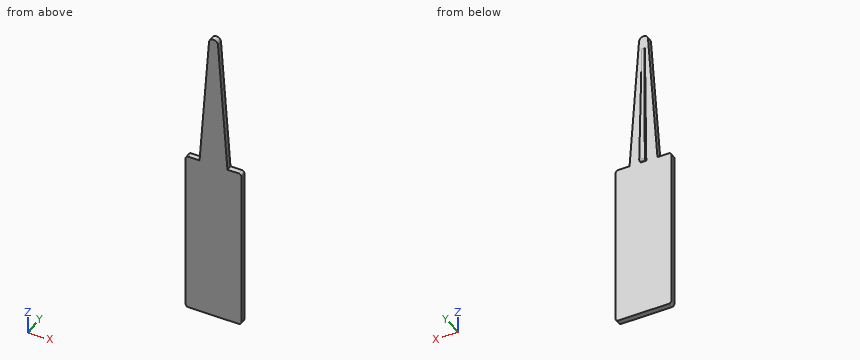
from build123d import *

# Parameters (mm, degrees)
BOSS_EXTRUDE1_DEPTH = 2
FILLET2_R           = 1
FILLET3_R           = 1
FILLET4_R           = 1
FILLET5_R           = 1
BOSS_EXTRUDE2_DEPTH = 1
DRAFT1_ANGLE        = -1
FILLET7_R           = 0.5


with BuildPart() as part:
    # Sketch1 → Boss-Extrude1 (new body)
    with BuildSketch(Plane(origin=(0, 0, 0), x_dir=(1, 0, 0), z_dir=(0, 1, 0))):
        with BuildLine():
            Line((0, 0), (20, 0))
            Line((20, 0), (20, -60))
            Line((20, -60), (15, -60))
            Line((15, -60), (11.6, -108.508220533))
            ThreePointArc((11.6, -108.508220533), (10, -110), (8.4, -108.508220533))
            Line((8.4, -108.508220533), (5, -60))
            Line((5, -60), (0, -60))
            Line((0, -60), (0, 0))
        make_face()
    extrude(amount=BOSS_EXTRUDE1_DEPTH)

    # Fillet2
    fillet2_edges = [part.edges().sort_by_distance(p)[0] for p in [
        (0, 1, 0),
    ]]
    fillet(fillet2_edges, radius=FILLET2_R)

    # Fillet3
    fillet3_edges = [part.edges().sort_by_distance(p)[0] for p in [
        (20, 1, 60),
    ]]
    fillet(fillet3_edges, radius=FILLET3_R)

    # Fillet4
    fillet4_edges = [part.edges().sort_by_distance(p)[0] for p in [
        (20, 1, 0),
    ]]
    fillet(fillet4_edges, radius=FILLET4_R)

    # Fillet5
    fillet5_edges = [part.edges().sort_by_distance(p)[0] for p in [
        (0, 1, 60),
    ]]
    fillet(fillet5_edges, radius=FILLET5_R)

    # Sketch5 → Boss-Extrude2 (add)
    with BuildSketch(Plane(origin=(0, 2, 0), x_dir=(1, 0, 0), z_dir=(0, 1, 0))):
        Polygon((11, -60), (9, -60), (9.5, -105), (10.5, -105), align=None)
    extrude(amount=BOSS_EXTRUDE2_DEPTH)

    # Draft1
    draft1_faces = [part.faces().sort_by_distance(p)[0] for p in [
        (10, 3, 80),
    ]]
    draft(draft1_faces, Plane(origin=(11, 3, 60), x_dir=(-1, 0, 0), z_dir=(0, 0, -1)), DRAFT1_ANGLE)

    # Fillet7
    fillet7_edges = [part.edges().sort_by_distance(p)[0] for p in [
        (10, 3, 60),
    ]]
    fillet(fillet7_edges, radius=FILLET7_R)


solid = part.part
Read the model definition and answer for the solid it produces. Units are mm, in the model's axes. Give positions to 0.01 mm unless a question says otherwise; leave off trailing zeros. Write each loop counter-clockwise with the first axis right and the second up, starting at its lowest first coordinate (ties: lowest second). Pieces come first, ordered by that corner, then holes. Notation, with made-up numbers: (88.5, 9.5) - (108.5, 9.5) arc R23 cw to (108.5, 48.5) - close; hole circle Ø10 at (-10.5, -17.75). An arc over 180 degrees is marked (long way). Return JSON: item names as keys, results as strings.
Q1. A cutting plane is placed at B-B, the plane z = 55. Determine the outline of the cut face in (x, y), and give its area (3 significant figures).
Reply:
{"outline": "(0, 0) - (20, 0) - (20, 2) - (0, 2) - close", "area": "40.0 mm²"}
Q2. A cutting plane is placed at A-A, the plane y = 0.9. Determine the outline of the cut face in (x, z).
Reply:
{"outline": "(0, 1) arc R1 ccw to (1, 0) - (19, 0) arc R1 ccw to (20, 1) - (20, 59) arc R1 ccw to (19, 60) - (15, 60) - (11.6, 108.51) arc R1.6 ccw to (8.4, 108.51) - (5, 60) - (1, 60) arc R1 ccw to (0, 59) - close"}
Q3. Consider line 1 along Y through (x, z) = (6.5, 18.5); line 2 along Z through (x, y) = (15.5, 0.8); line 3 along X through (y, z) = (2.65, 76). Determine where each line is inside the solid, lowest interval first. Write a range as [from, to].
Reply:
{"line 1": "[0, 2]", "line 2": "[0, 60]", "line 3": "[9.18, 10.82]"}
Q4. Given P1, Ø2, axis at x = 8, z = 89.5, coming from the +Y side; P2, Ø1.6, axis at x = 3, y = 1, coming from the +Z side; P3, Ø0.5, axis at x = 10, y = 2.5, coming from the -Z side, each flat-ended and moving along its own axis, determine where each tip first touches the part or whether it passes through.
Reply:
{"P1": "y = 2", "P2": "z = 60", "P3": "z = 60"}
Q5. A cutting plane is placed at D-D, the plane z = 92. Determine the outline of the cut face in (x, y).
Reply:
{"outline": "(7.24, 0) - (12.76, 0) - (12.76, 2) - (10.64, 2) - (10.64, 2.44) - (9.36, 2.44) - (9.36, 2) - (7.24, 2) - close"}
Q6. A cutting plane is placed at C-C, the plane x = 12.75. Determine the outline of the cut face in (y, z), and give its area (3 significant figures).
Reply:
{"outline": "(0, 0) - (2, 0) - (2, 92.1) - (0, 92.1) - close", "area": "184 mm²"}
